The listing builds one solid part. Answer for the finished solid, in the listing's coordinates (mm). A direction names the side the tool comes from. Give positions to 0.01 mm unless a question says otherwise; leave off trailing zeros. Write each loop counter-clockwise with the first axis right and the second up, starting at its lowest first coordinate (ties: lowest second). Pieces come first, ordered by that corner, then holes. Notation, with made-up numbers: (-0.75, -31) - (29.25, -31) arc R20 cw to (29.25, -3) - close; hole circle Ø4 at (80, 24.25). An arc over 180 degrees is marked (long way). Answer in a Markdown table with one row per item. Add a question column.
from build123d import *

# Parameters (mm, degrees)
SKETCH1_W               = 189.5
SKETCH1_H               = 111.6
BOSS_EXTRUDE1_DEPTH     = 80
SKETCH3_R               = 8.15
CUT_EXTRUDE2_DEPTH      = 40
SKETCH4_R               = 10.3
CUT_EXTRUDE3_DEPTH      = 40
CUT_EXTRUDE1_START      = -189.5
CUT_EXTRUDE1_DEPTH      = 189.5
CUT_EXTRUDE5_START      = -10
SKETCH5_R               = 83.637561864
CUT_EXTRUDE5_DEPTH      = 196.625563976
SKETCH6_R               = 2
CUT_EXTRUDE6_DEPTH      = 15
CUT_EXTRUDE7_DEPTH      = 142.983674128
CUT_EXTRUDE7_DEPTH_BACK = 142.983674128
SKETCH7_R               = 1


# Read off the part's stored shape, not the designer's step: Cut-Extrude1
with BuildPart() as part:
    # Sketch1 → Boss-Extrude1 (new body)
    with BuildSketch(Plane(origin=(0, 0, 0), x_dir=(1, 0, 0), z_dir=(0, 1, 0))):
        with Locations((26.340909091, -2.05)):
            Rectangle(SKETCH1_W, SKETCH1_H)
    extrude(amount=BOSS_EXTRUDE1_DEPTH)

    # Sketch3 → Cut-Extrude2 (cut)
    with BuildSketch(Plane.XY.offset(57.85)):
        with Locations((-6.709090909, 45)):
            Circle(SKETCH3_R)
        with Locations((44.290909091, 45)):
            Circle(SKETCH3_R)
        with Locations((95.290909091, 45)):
            Circle(SKETCH3_R)
    extrude(amount=-CUT_EXTRUDE2_DEPTH, mode=Mode.SUBTRACT)

    # Sketch4 → Cut-Extrude3 (cut)
    with BuildSketch(Plane(origin=(0, 0, -53.75), x_dir=(-1, 0, 0), z_dir=(0, 0, -1))):
        with Locations((-18.790909091, 45)):
            Circle(SKETCH4_R)
    extrude(amount=-CUT_EXTRUDE3_DEPTH, mode=Mode.SUBTRACT)

    # Cut-Extrude1 outline → Cut-Extrude1 (cut)
    with BuildSketch(Plane.ZY.offset(68.409090909).offset(CUT_EXTRUDE1_START)):
        with BuildLine():
            Line((-53.75, 55), (-48.75, 55))
            ThreePointArc((-48.75, 55), (2.05, 4.2), (52.85, 55))
            Line((52.85, 55), (57.85, 55))
            Line((57.85, 55), (57.85, 80))
            Line((57.85, 80), (-53.75, 80))
            Line((-53.75, 80), (-53.75, 55))
        make_face()
    extrude(amount=CUT_EXTRUDE1_DEPTH, mode=Mode.SUBTRACT)

    # Sketch5 → Cut-Extrude5 (cut, through all)
    with BuildSketch(Plane.ZY.offset(68.409090909).offset(CUT_EXTRUDE5_START)):
        with Locations((5.899408019, 41.151011042)):
            Circle(SKETCH5_R)
    extrude(amount=-CUT_EXTRUDE5_DEPTH, mode=Mode.SUBTRACT)

    # Sketch6 → Cut-Extrude6 (cut)
    with BuildSketch(Plane.XZ):
        with Locations(Location((-63.409090909, 42.85, 0), (0, 0, 270))):
            Circle(SKETCH6_R)
        with Locations(Location((-63.409090909, -38.75, 0), (0, 0, 270))):
            Circle(SKETCH6_R)
    extrude(amount=-CUT_EXTRUDE6_DEPTH, mode=Mode.SUBTRACT)

    # Sketch7 → Cut-Extrude7 (cut, two sides: drawn at the far end of the back side and taken through both)
    with BuildSketch(Plane.XY.offset(57.85).offset(-CUT_EXTRUDE7_DEPTH_BACK)):
        with Locations((-63.409090909, 50)):
            Circle(SKETCH7_R)
    extrude(amount=CUT_EXTRUDE7_DEPTH + CUT_EXTRUDE7_DEPTH_BACK, mode=Mode.SUBTRACT)


solid = part.part
1. Given pin 1 Ø3 at (x, z) = (-63.41, 42.85) entering from +Y; pin 2 Ø2.5 at (x, z) = (-63.41, -38.75) entering from -Y; pin 3 Ø3 at (x, z) = (-63.5, 43.5) entering from -Y; pin 4 Ø3 at (x, z) = (-61.5, 46.5) entering from +Y, each flat-ended and moving along its own axis, determine where each tip first touches the part or whether it passes through.
2. Section D-D (x = -60) is taken. Give the vertices of the cut face in (y, z).
3. Section A-A (y = 13) is taken. Give the vertices of the cut face in (x, z), and give its area (3 significant figures).
4. Section C-C (y = 50) is taken. Give the vertices of the cut face in (x, z).
5. The mould has two halves that part along Y. Classify faces 1 (the face through (-63, 55, -51)), 2 (the face through (-62.87, 50.84, -51.11)), 3 (the face through (-63, 0, 1)), 4 (the face through (-62.87, 50.84, 55.13)): +Y half, -Y half, draft (parallel to the pull), parting line (faces both ways), or undercut.
6. Straight lines are drawn through the part: L1, parallel to Z at x = -64.75, y = 11; L2, parallel to Z at x = -63.75, y = 10; L3, parallel to X at y = 50, z = -50.55. For each, find the intervals that lie inside material, in ascending order. Write a range as [from, to].
7. A tool of negligible diameter and unlimited length cuts with its end or side. For faces 5 (the face through (-63, 15, -39)), 6 (the face through (-63.339, 4.212, 0.933)), from which of +Z, -Z, +X, -X, +Y, -Y can it reach the whole face along a straight path? Write none if from no direction.
8. Section B-B (y = 39.5) is taken. Give the vertices of the cut face in (x, z), and give its area (3 significant figures).
Geometry check:
| question | item | result |
|---|---|---|
| 1 | pin 1 | y = 26.87 |
| 1 | pin 2 | y = 15 |
| 1 | pin 3 | y = 0 |
| 1 | pin 4 | y = 33.34 |
| 2 | outline | (0, -53.75) - (55, -53.75) - (55, -48.75) arc R50.8 cw to (55, 52.85) - (55, 57.85) - (0, 57.85) - close |
| 3 | outline | (-68.41, -53.75) - (-58.41, -53.75) - (-58.41, -26.53) - (-68.41, -26.53) - close; (-68.41, 30.63) - (-58.41, 30.63) - (-58.41, 57.85) - (-68.41, 57.85) - close; hole circle Ø4 at (-63.41, -38.75); hole circle Ø4 at (-63.41, 42.85) |
| 3 | area | 519 mm² |
| 4 | outline | (-68.41, -53.75) - (-64.41, -53.75) - (-64.41, -48.5) - (-68.41, -48.5) - close; (-68.41, 52.6) - (-64.41, 52.6) - (-64.41, 57.85) - (-68.41, 57.85) - close; (-62.41, -53.75) - (-58.41, -53.75) - (-58.41, -48.5) - (-62.41, -48.5) - close; (-62.41, 52.6) - (-58.41, 52.6) - (-58.41, 57.85) - (-62.41, 57.85) - close |
| 5 | face 1 | +Y half |
| 5 | face 2 | undercut |
| 5 | face 3 | -Y half |
| 5 | face 4 | undercut |
| 6 | L1 | [-53.75, -40.23], [-37.27, -23.34], [27.44, 41.37], [44.33, 57.85] |
| 6 | L2 | [-53.75, -40.72], [-36.78, -21.52], [25.62, 40.88], [44.82, 57.85] |
| 6 | L3 | [-68.41, -64.41], [-62.41, -58.41] |
| 7 | face 5 | -Y |
| 7 | face 6 | +X, -X, +Y |
| 8 | outline | (-68.41, -53.75) - (-58.41, -53.75) - (-58.41, -46.33) - (-68.41, -46.33) - close; (-68.41, 50.43) - (-58.41, 50.43) - (-58.41, 57.85) - (-68.41, 57.85) - close |
| 8 | area | 148 mm² |
